Verification items for this drawing (mm, ordinates from the low corner). Give positions to 0.01 mm unless a question says otherwise; leave off trailing zeros. Loops run counter-clockwise (first coordinate to the right, second up) from the corner with the lowest first, then second, coordinate; pieces in that order, holes last. Notation, with made-up numbers: (-38.5, -4) -> (17.5, -4) arc R15 cw to (17.5, 25) -> close; hole circle Ø2 at (26, 25). An arc over 180 degrees is marked (long way). Write item = value, one per line.
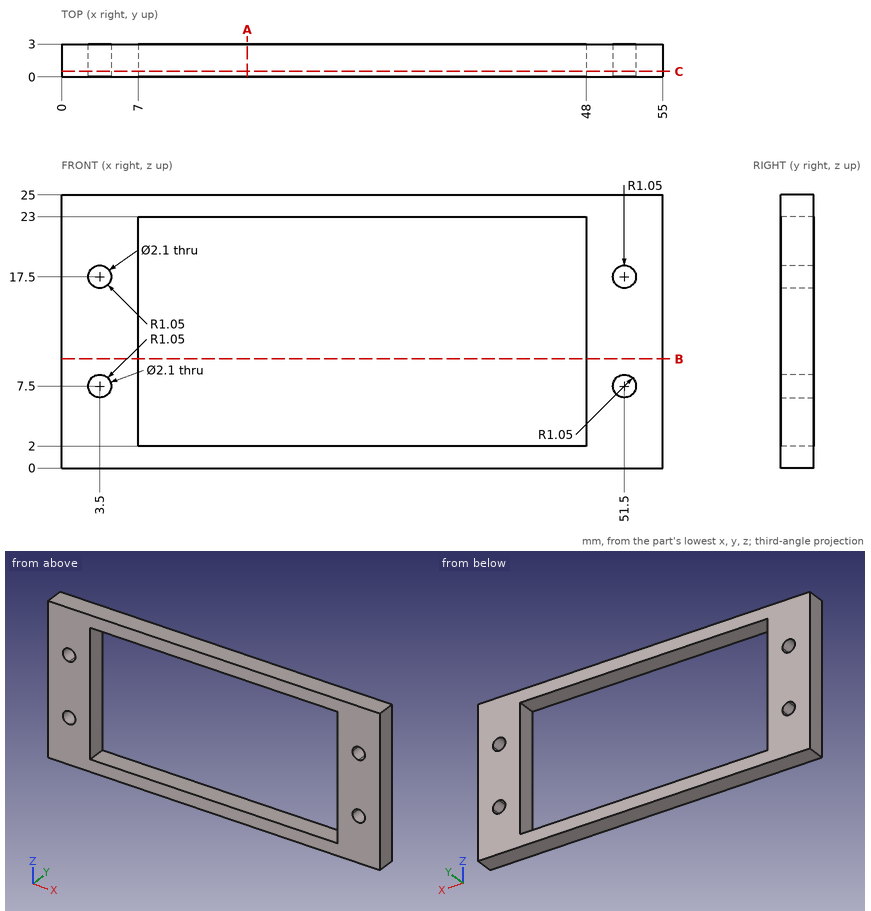
Item 1: Gauge pin test, flat end, axial feed: pin 1 (1.3 mm diameter, centred on x = 3.5, z = 17.5, fed in from -Y). Record the tip position at first contact, or that the pin passes through.
Answer:
pin_1 = through
Item 2: Section check C-C, the plane y = 0.5. Record the cut outline in (x, z).
Answer:
outline = (0, 0) -> (55, 0) -> (55, 25) -> (0, 25) -> close; hole circle Ø2.1 at (3.5, 7.5); hole circle Ø2.1 at (3.5, 17.5); hole (7, 2) -> (48, 2) -> (48, 23) -> (7, 23) -> close; hole circle Ø2.1 at (51.5, 7.5); hole circle Ø2.1 at (51.5, 17.5)
Item 3: Thickness scan on L1, parallel to Z at x = 3.5, y = 2.25; L2, parallel to X at y = 1.2, z = 17.5; L3, parallel to Z at x = 35, y = 2.1. Record the ranges inside material, lowest first. Write a range as [from, to].
Answer:
L1 = [0, 6.45], [8.55, 16.45], [18.55, 25]
L2 = [0, 2.45], [4.55, 7], [48, 50.45], [52.55, 55]
L3 = [0, 2], [23, 25]
Item 4: Section check A-A, the plane x = 17. Record the cut outline in (y, z), plus the area to 3 significant figures.
Answer:
outline = (0, 0) -> (3, 0) -> (3, 2) -> (0, 2) -> close; (0, 23) -> (3, 23) -> (3, 25) -> (0, 25) -> close
area = 12.0 mm^2
Item 5: Section check B-B, the plane z = 10. Record the cut outline in (x, y), plus the area to 3 significant figures.
Answer:
outline = (0, 0) -> (7, 0) -> (7, 3) -> (0, 3) -> close; (48, 0) -> (55, 0) -> (55, 3) -> (48, 3) -> close
area = 42.0 mm^2
